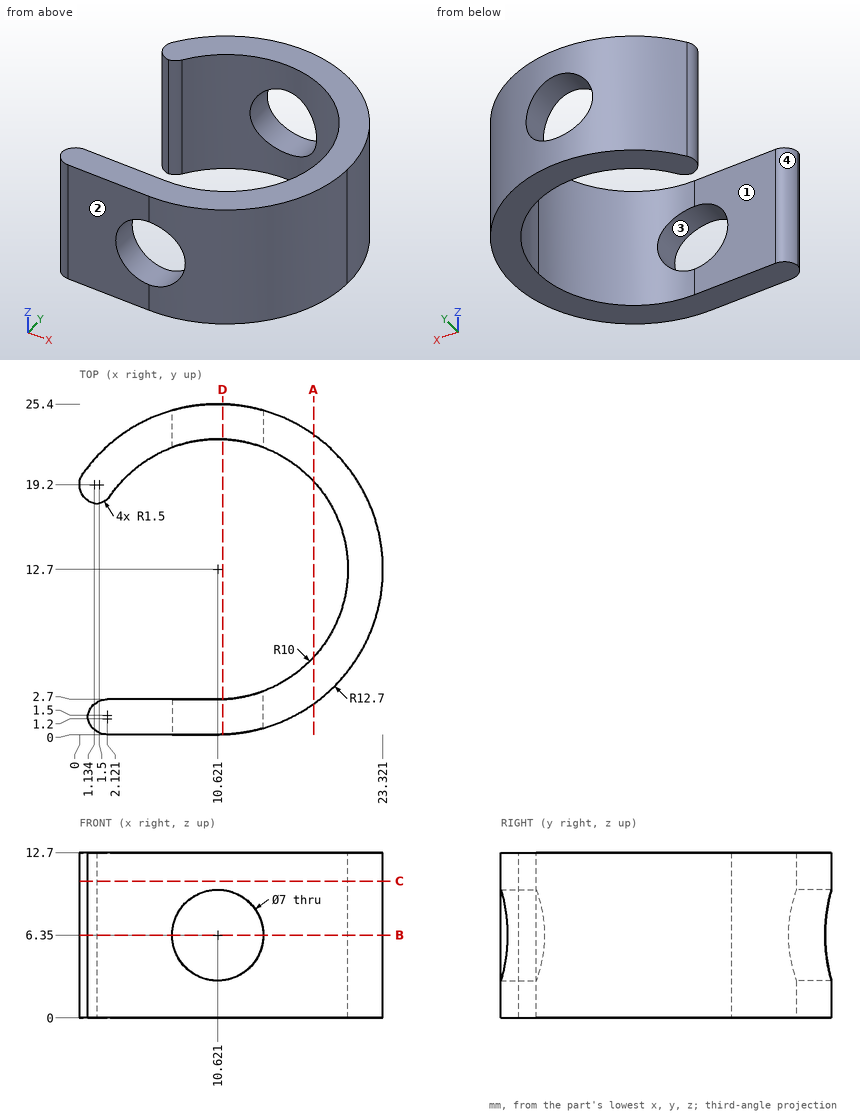
Can you work these out from the drawing? Everything is in mm from the part's minimum corner. Coordinates: 2 decimals unless noted, no trailing zeros. Order: outer loops, then holes, each group sorted by start corner. A loop starts at its lowest first (then second) coordinate and runs counter-clockwise, first axis right, second up. Notation, with made-up numbers: M -6,-26.5 L 13,-26.5 A19 ccw 13,-20.5 Z; hole C -23.5,65 d5. An arc over 180 degrees is marked long. Answer as CSV lines item,"result". Start each with the question number.
1. I want a section at C-C, the plane z = 10.5. Write out the boundary of the cut face in (x, y).
2. I want a section at B-B, the plane z = 6.35. Write out the boundary of the cut face in (x, y), and give its area (3 significant figures).
3. For pin 1 (1.5 mm diameter, centred on y = 8.5, z = 10, fed in from -X); pin 2 (6.5 mm diameter, centred on x = 10.62, z = 6.35, fed in from +Y); pin 3 (10 mm diameter, centred on x = 15.5, y = 17.5, fed in from -Z); pin 4 (3 mm diameter, centred on x = 18.5, z = 6, fed in from +Y), each with a flat end and sliding along its axis, tell me the tip position at first contact or that it passes through.
4. We'd pull the mould along Y, two halves only. Please class the marked faces 1, 2, 3 and 4: released by +Y, released by -Y, zero draft, split by the parting line, or undercut.
5. I want a section at A-A, the plane x = 18. Write out the boundary of the cut face in (y, z).
6. I need wall thicknesses on line 1 (Y direction, x = 16.25, z = 0.5) (1 decimal); line 2 (Y direction, x = 4.5, z = 12); line 3 (X direction, y = 19.25, z = 3) (1 decimal). Which ranges of each line are inside material? Lowest first, please. Write a range as [from, to].
7. I want a section at D-D, the plane x = 11. Write out the boundary of the cut face in (y, z), and give its area (3 significant figures).
Recorded:
1,outline,"M 0.28,20.07 A1.5 ccw 1.32,17.71 A1.5 ccw 2.37,18.35 A10 cw long 10.62,2.7 L 2.12,2.7 A1.5 ccw 0.63,1.35 A1.5 ccw 2.12,0 L 10.62,0 A12.7 ccw long Z"
2,outline,"M 0.28,20.07 A1.5 ccw 1.32,17.71 A1.5 ccw 2.37,18.35 A10 cw 7.12,22.07 L 7.12,24.91 A12.7 ccw Z; M 0.63,1.35 A1.5 ccw 2.12,0 L 7.12,0 L 7.12,2.7 L 2.12,2.7 A1.5 ccw Z; M 14.12,0.49 A12.7 ccw 14.12,24.91 L 14.12,22.07 A10 cw 14.12,3.33 Z"
2,area,"116 mm2"
3,pin 1,"stops at x = 19.31"
3,pin 2,"passes through"
3,pin 3,"stops at z = 0"
3,pin 4,"stops at y = 23.68"
4,face 1,"undercut"
4,face 2,"released by -Y"
4,face 3,"zero draft"
4,face 4,"undercut"
5,outline,"M 2.36,0 L 5.95,0 L 5.95,12.7 L 2.36,12.7 Z; M 19.45,0 L 23.04,0 L 23.04,12.7 L 19.45,12.7 Z"
6,line 1,"y = [1.3, 4.4], [21, 24.1]"
6,line 2,"y = [0, 2.7], [20.61, 23.83]"
6,line 3,"x = [0, 3.1], [18.2, 21.5]"
7,outline,"M 0.01,0 L 2.71,0 L 2.71,2.87 L 0.01,2.87 Z; M 0.01,9.83 L 2.71,9.83 L 2.71,12.7 L 0.01,12.7 Z; M 22.69,0 L 25.39,0 L 25.39,2.87 L 22.69,2.87 Z; M 22.69,9.83 L 25.39,9.83 L 25.39,12.7 L 22.69,12.7 Z"
7,area,"31.0 mm2"
